Read the model definition and answer for the solid it produces. Units are mm, in the model's axes. Face numbers are marked on the shaded views. A direction names the side the tool comes from. Round coordinates to 2 decimals unless told otherwise and drop trailing zeros. Write each loop counter-clockwise with the first axis right and the second up, starting at its lowest first coordinate (ties: lowest second). Pieces come first, ordered by that corner, then holes. Notation, with made-up numbers: (-6.5, 43.25) - (33.5, 43.25) arc R26 cw to (33.5, 61.25) - close; hole circle Ø10 at (14, 70.25). An arc over 180 degrees is marked (long way). Use one line per item in the form item = value. Start each with the question number.
1) The part is cut by section B-B, the plane y = 4.75. Give the vertices of the cut face in (x, z), plus the area to 3 significant figures.
2) The part is cut by section D-D, the plane z = 9.5. Give the vertices of the cut face in (x, y).
3) The part is cut by section C-C, the plane x = 37. Give the vertices of the cut face in (y, z).
4) Consider line 1 along Z through (x, y) = (22, 9.5); line 2 along X through (y, z) = (11, 1.5); line 3 along X through (y, z) = (8.75, -0.5). Determine where each line is inside the solid, lowest interval first. Write a range as from..to.
5) The part is cut by section A-A, the plane z = -1.5. Give the vertices of the cut face in (x, y), plus the area to 3 significant figures.
6) For the marked faces 1 and 2, determine the directions among +Z, -Z, +X, -X, +Y, -Y from which every point of the face is accessible in a straight line to the end or side of a thin tool.
7) Each of these flat-tipped pins is pushed along its axis until it touches: pin 1 (8 mm diameter, centred on x = 12.5, z = 3, fed in from -Y); pin 2 (1 mm diameter, centred on y = 15.5, z = 1.5, fed in from +X); pin 3 (6 mm diameter, centred on x = 12.5, y = 13.5, fed in from +Z); pin 4 (0.9 mm diameter, centred on y = 9, z = -1.5, fed in from -X). Where does it stop, or does it pass through?
from build123d import *

# Parameters (mm, degrees)
BOSS_EXTRUDE1_DEPTH = 20
SKETCH2_W           = 5
SKETCH2_H           = 5
CUT_EXTRUDE1_DEPTH  = 10


with BuildPart() as part:
    # Sketch1 → Boss-Extrude1 (new body)
    with BuildSketch(Plane(origin=(0, 0, 0), x_dir=(1, 0, 0), z_dir=(0, 1, 0))):
        Polygon((0, 0), (0, 3), (50, 3), (59.984585881, -11.976917065), (56.379037438, -11.976917065), (48.39444645, 0), align=None)
    extrude(amount=BOSS_EXTRUDE1_DEPTH)

    # Sketch2 → Cut-Extrude1 (cut)
    with BuildSketch(Plane(origin=(0, 0, -3), x_dir=(-1, 0, 0), z_dir=(0, 0, -1))):
        with Locations((-2.5, 10)):
            Rectangle(SKETCH2_W, SKETCH2_H)
    extrude(amount=-CUT_EXTRUDE1_DEPTH, mode=Mode.SUBTRACT)


solid = part.part
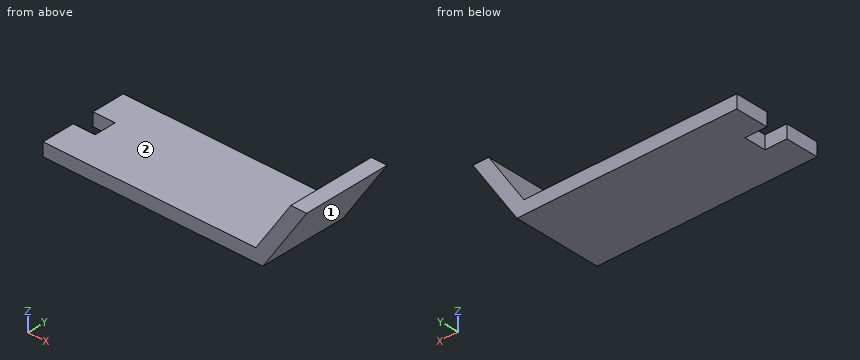
Geometry results:
q1.outline = (0, -3) - (50, -3) - (59.98, 11.98) - (56.38, 11.98) - (48.39, 0) - (0, 0) - close
q1.area = 196 mm2
q2.outline = (54.73, 0) - (58.33, 0) - (58.33, 20) - (54.73, 20) - close
q3.outline = (0, -3) - (20, -3) - (20, 0) - (0, 0) - close
q4.line_1 = -3..0
q4.line_2 = 49.39..53
q4.line_3 = 5..51.67
q5.outline = (0, 0) - (51, 0) - (51, 20) - (0, 20) - (0, 12.5) - (5, 12.5) - (5, 7.5) - (0, 7.5) - close
q5.area = 995 mm2
q6.face_1 = -Z, +X, +Y, -Y
q6.face_2 = +Z, -X, +Y, -Y
q7.pin_1 = 0
q7.pin_2 = 53.33
q7.pin_3 = 0
q7.pin_4 = 5
